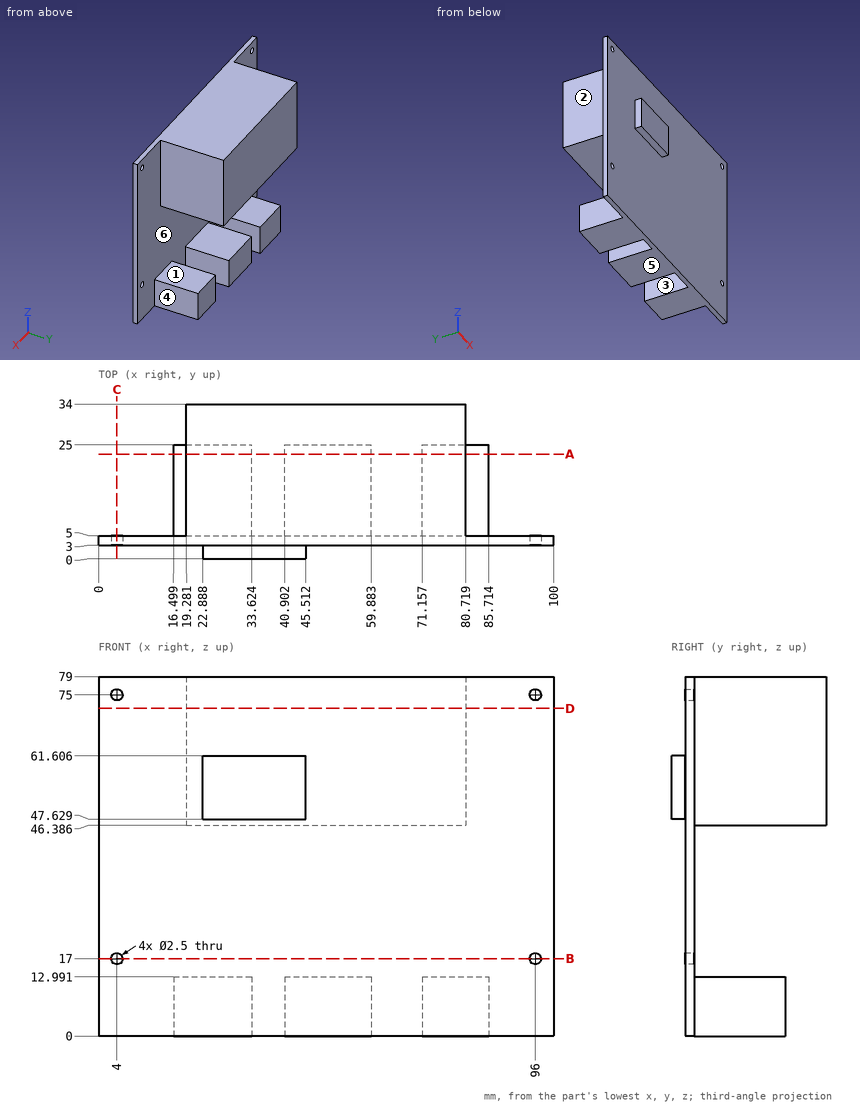
Geometry check sheet. Reference: drawing and pictorial views, mm from the part's lowest x, y, z. A direction names the side the tool comes from. Coordinates: 2 decimals unless noted, no trailing zeros. Order: outer loops, then holes, each group sorted by start corner. A loop starts at its lowest first (then second) coordinate and runs counter-clockwise, first axis right, second up.
Item 1: Section check C-C, the plane x = 4. Enter the section's corners in (y, z).
Filled in:
outline: (3, 0) - (5, 0) - (5, 15.75) - (3, 15.75) - close; (3, 18.25) - (5, 18.25) - (5, 73.75) - (3, 73.75) - close; (3, 76.25) - (5, 76.25) - (5, 79) - (3, 79) - close
Item 2: Section check A-A, the plane y = 23. Enter the section's corners in (x, z) (1 decimal), then the cut area to 3 significant figures.
Filled in:
outline: (16.5, 0) - (33.6, 0) - (33.6, 13) - (16.5, 13) - close; (19.3, 46.4) - (80.7, 46.4) - (80.7, 79) - (19.3, 79) - close; (40.9, 0) - (59.9, 0) - (59.9, 13) - (40.9, 13) - close; (71.2, 0) - (85.7, 0) - (85.7, 13) - (71.2, 13) - close
area: 2,660 mm2
Item 3: Access from +Z, -Z, +X, -X, +Y, -Y to the whole of each face (thin tool, end or side, straight path). Record for the marked faces 1, 2 and 3.
Filled in:
face 1: +X, -X, +Y
face 2: +Z, -X, +Y
face 3: -Z, +Y
Item 4: Material ranges on L1, parallel to X at y = 4, z = 17; L2, parallel to X at y = 14, z = 10.5; L3, parallel to Z at x = 96, y = 3.85, recorded low to high.
Filled in:
L1: x = 0 to 2.75, 5.25 to 94.75, 97.25 to 100
L2: x = 16.5 to 33.62, 40.9 to 59.88, 71.16 to 85.71
L3: z = 0 to 15.75, 18.25 to 73.75, 76.25 to 79
Item 5: Release check for a two-part mould opening along Z. For the marked faces 4, 5 and 6 record: +Z half, -Z half, draft (parallel to the pull), parting line (faces both ways), or undercut.
Filled in:
face 4: draft
face 5: -Z half
face 6: undercut
Item 6: Depth check by flat-ended pin: pin 1 (8 mm diameter, centred on x = 16, y = 28.5, fed in from +Z); pin 2 (1.5 mm diameter, centred on y = 1, z = 57.5, fed in from +X); pin 3 (4 mm diameter, centred on x = 24, z = 6.5, fed in from +Y); pin 4 (8.5 mm diameter, centred on y = 14.5, z = 63, fed in from -X). Enter the tip coordinate at first touch or a pass-through.
Filled in:
pin 1: stops at z = 79
pin 2: stops at x = 45.51
pin 3: stops at y = 25
pin 4: stops at x = 19.28
Item 7: Section check D-D, the plane z = 72. Enter the section's corners in (x, y), then the cut area to 3 significant figures.
Filled in:
outline: (0, 3) - (100, 3) - (100, 5) - (80.72, 5) - (80.72, 34) - (19.28, 34) - (19.28, 5) - (0, 5) - close
area: 1,980 mm2
Item 8: Section check B-B, the plane z = 17. Enter the section's corners in (x, y).
Filled in:
outline: (0, 3) - (2.75, 3) - (2.75, 5) - (0, 5) - close; (5.25, 3) - (94.75, 3) - (94.75, 5) - (5.25, 5) - close; (97.25, 3) - (100, 3) - (100, 5) - (97.25, 5) - close
